```python
from build123d import *

# Parameters (mm, degrees)
ALUMINUM_PLATE_DEPTH            = 3.175
LPATTERN1_COUNT                 = 2
LPATTERN1_PITCH                 = 35
LPATTERN1_COUNT_DIR2            = 2
LPATTERN1_PITCH_DIR2            = 77
CIRPATTERN1_COUNT               = 4
TAP_DRILL_FOR_M5X0_8_TAP1_D     = 4.2
TAP_DRILL_FOR_M5X0_8_TAP1_DEPTH = 25.4
TAP_DRILL_FOR_M5X0_8_TAP1_TIP   = 1.2618073
TAP_DRILL_FOR_8_32_TAP1_D       = 3.4544
TAP_DRILL_FOR_8_32_TAP1_DEPTH   = 12.7
TAP_DRILL_FOR_8_32_TAP1_TIP     = 1.037806461
CUT_EXTRUDE1_DEPTH              = 3.175
CIRPATTERN3_COUNT               = 4
TAP_DRILL_FOR_6_32_TAP1_D       = 2.7051
TAP_DRILL_FOR_6_32_TAP1_DEPTH   = 12.7
TAP_DRILL_FOR_6_32_TAP1_TIP     = 0.81269403


with BuildPart() as part:
    # Sketch2 → Aluminum plate (new body)
    with BuildSketch(Plane(origin=(0, 0, 0), x_dir=(1, 0, 0), z_dir=(0, 1, 0))):
        with BuildLine():
            Line((58.024404898, -30.931736602), (-20.876528813, -30.930973959))
            ThreePointArc((-20.876528813, -30.930973959), (-24.412048563, -29.466473691), (-25.876480484, -25.93092563))
            Line((-25.876480484, -25.93092563), (-25.875595093, 65.669074365))
            ThreePointArc((-25.875595093, 65.669074365), (-24.411094826, 69.204594116), (-20.875546764, 70.669026036))
            Line((-20.875546764, 70.669026036), (58.024501561, 70.668263401))
            ThreePointArc((58.024501561, 70.668263401), (61.560004224, 69.20378022), (63.024453231, 65.668263401))
            Line((63.024453231, 65.668263401), (63.024453227, -25.931736603))
            ThreePointArc((63.024453227, -25.931736603), (61.559970046, -29.467287596), (58.024404898, -30.931736602))
        make_face()
        Polygon((40.164453228, -4.2611466), (-3.015546772, -4.261146598), (-3.01554677, 38.918853402), (40.16445323, 38.9188534), align=None, mode=Mode.SUBTRACT)
    extrude(amount=ALUMINUM_PLATE_DEPTH)

    # Sketch12 → Tap Drill for M3x0.5 Tap1 (revolve, cut)
    with BuildSketch(Plane(origin=(-19.925892409, 3.175, -34.909619628), x_dir=(0, 0, 1), z_dir=(1, 0, 0))):
        Polygon((0, 0), (0, 26.151075774), (1.25, 25.4), (1.25, 0), align=None)
    tap_drill_for_m3x0_5_tap1 = revolve(axis=Axis((-19.925892409, 9.525, -34.909619628), (0, -1, 0)), mode=Mode.SUBTRACT)

    # LPattern1: Tap Drill for M3x0.5 Tap1 2 × 2
    with Locations(*[(j * LPATTERN1_PITCH_DIR2, 0, i * LPATTERN1_PITCH) for i in range(LPATTERN1_COUNT) for j in range(LPATTERN1_COUNT_DIR2) if (i, j) != (0, 0)]):
        add(tap_drill_for_m3x0_5_tap1, mode=Mode.SUBTRACT)

    # Sketch14 → Tap Drill for M3x0.5 Tap2 (revolve, cut)
    with BuildSketch(Plane(origin=(42.384453228, 3.175, -17.329161252), x_dir=(0, 0, 1), z_dir=(1, 0, 0))):
        Polygon((0, 0), (0, 26.151075774), (1.25, 25.4), (1.25, 0), align=None)
    tap_drill_for_m3x0_5_tap2 = revolve(axis=Axis((42.384453228, 9.525, -17.329161252), (0, -1, 0)), mode=Mode.SUBTRACT)

    # CirPattern1: Tap Drill for M3x0.5 Tap2 ×4 about axis
    cirpattern1_axis = Axis((18.574453229, 0, -17.328853401), (0, 1, 0))
    for i in range(1, CIRPATTERN1_COUNT):
        add(tap_drill_for_m3x0_5_tap2.rotate(cirpattern1_axis, i * 360 / CIRPATTERN1_COUNT), mode=Mode.SUBTRACT)

    # Tap Drill for M5x0.8 Tap1
    with Locations(Plane.XZ):
        with Locations((-19.525700823, -54.730512991), (56.674299173, -54.729776455), (56.67357614, 20.073223545), (-19.526423857, 20.072487009)):
            Hole(TAP_DRILL_FOR_M5X0_8_TAP1_D / 2, depth=TAP_DRILL_FOR_M5X0_8_TAP1_DEPTH)
            with Locations((0, 0, -(TAP_DRILL_FOR_M5X0_8_TAP1_DEPTH + TAP_DRILL_FOR_M5X0_8_TAP1_TIP / 2))):  # 118° drill point
                Cone(0, TAP_DRILL_FOR_M5X0_8_TAP1_D / 2, TAP_DRILL_FOR_M5X0_8_TAP1_TIP, mode=Mode.SUBTRACT)

    # Tap Drill for _8-32 Tap1
    with Locations(Plane(origin=(0, 3.175, 0), x_dir=(-1, 0, 0), z_dir=(0, 1, 0))):
        with Locations((-2.699395239, -64.668798164), (-34.449395238, -64.668491274)):
            Hole(TAP_DRILL_FOR_8_32_TAP1_D / 2, depth=TAP_DRILL_FOR_8_32_TAP1_DEPTH)
            with Locations((0, 0, -(TAP_DRILL_FOR_8_32_TAP1_DEPTH + TAP_DRILL_FOR_8_32_TAP1_TIP / 2))):  # 118° drill point
                Cone(0, TAP_DRILL_FOR_8_32_TAP1_D / 2, TAP_DRILL_FOR_8_32_TAP1_TIP, mode=Mode.SUBTRACT)

    # Sketch24 → Cut-Extrude1 (cut)
    with BuildSketch(Plane(origin=(0, 3.175, 0), x_dir=(1, 0, 0), z_dir=(0, 1, 0))):
        with BuildLine():
            Line((21.16445323, 40.9188534), (21.16445323, 44.8563534))
            ThreePointArc((21.16445323, 44.8563534), (21.750239668, 46.270566962), (23.16445323, 46.8563534))
            Line((23.16445323, 46.8563534), (46.101953228, 46.8563534))
            ThreePointArc((46.101953228, 46.8563534), (47.516166791, 46.270566962), (48.101953228, 44.8563534))
            Line((48.101953228, 44.8563534), (48.101953228, 21.9188534))
            ThreePointArc((48.101953228, 21.9188534), (47.516166791, 20.504639837), (46.101953228, 19.9188534))
            Line((46.101953228, 19.9188534), (42.164453228, 19.9188534))
            ThreePointArc((42.164453228, 19.9188534), (40.750239666, 19.333066962), (40.164453228, 17.9188534))
            Line((40.164453228, 17.9188534), (40.164453228, 17.3288534))
            Line((40.164453228, 17.3288534), (18.57445323, 38.9188534))
            Line((18.57445323, 38.9188534), (19.16445323, 38.9188534))
            ThreePointArc((19.16445323, 38.9188534), (20.578666793, 39.504639837), (21.16445323, 40.9188534))
        make_face()
    cut_extrude1 = extrude(amount=-CUT_EXTRUDE1_DEPTH, mode=Mode.SUBTRACT)

    # CirPattern3: Cut-Extrude1 ×4 about axis
    cirpattern3_axis = Axis((18.574453229, 0, -17.328853401), (0, 1, 0))
    for i in range(1, CIRPATTERN3_COUNT):
        add(cut_extrude1.rotate(cirpattern3_axis, i * 360 / CIRPATTERN3_COUNT), mode=Mode.SUBTRACT)

    # Tap Drill for _6-32 Tap1
    with Locations(Plane(origin=(0, 3.175, 0), x_dir=(-1, 0, 0), z_dir=(0, 1, 0))):
        with Locations((-11.032976674, 17.431282391), (-26.114226674, 17.431282391)):
            Hole(TAP_DRILL_FOR_6_32_TAP1_D / 2, depth=TAP_DRILL_FOR_6_32_TAP1_DEPTH)
            with Locations((0, 0, -(TAP_DRILL_FOR_6_32_TAP1_DEPTH + TAP_DRILL_FOR_6_32_TAP1_TIP / 2))):  # 118° drill point
                Cone(0, TAP_DRILL_FOR_6_32_TAP1_D / 2, TAP_DRILL_FOR_6_32_TAP1_TIP, mode=Mode.SUBTRACT)


solid = part.part
```
Work out the finished part from the listing and answer in its coordinate system (mm). Give positions to 0.01 mm unless a question says otherwise; leave off trailing zeros. Loops run counter-clockwise (first coordinate to the right, second up) from the corner with the lowest first, then second, coordinate; pieces in that order, holes last. Notation, with made-up numbers: M -15,48 L 24,48 A29 ccw 24,69 Z; hole C 81.5,53 d6. An arc over 180 degrees is marked long. One line per item, written item: value. Start each with the question number.
1. Determine the mould class of faces 1 (the face through (-24.45, 1.565, -69.166)), 2 (the face through (10.857, 1.565, 18.772)), 3 (the face through (63.024, 2, -21)), 4 (the face through (15.984, 2, -43)) for opening direction Z: released by +Z, released by -Z, zero draft, split by the parting line, or undercut.
2. Find the intervals of material crossed by probe 1 along Z at (x, y) = (-7, 0.65); probe 2 along X at (y, z) = (2.1, -28); probe 3 along Z at (x, y) = (18, 1.55), in increasing order.
3. Each of these flat-tipped pins is pushed along its axis until it touches: P1, Ø2, axis at x = 34.45, z = -64.67, coming from the +Y side; P2, Ø5.5, axis at x = 56.67, z = 20.07, coming from the +Y side (3 decimals). Where does it stop, or does it pass through?
4. Find section C-C (y = 0.7). State how many separate pieces and enclosed holes the cut face has, and give its area (3 significant figures).
5. Find section A-A (z = -30). Give the vertices of the cut face in (x, y) (3 decimals), and give its area (3 significant figures).
Reported:
1. face 1: released by -Z
1. face 2: undercut
1. face 3: zero draft
1. face 4: undercut
2. probe 1: z = -70.67 to -46.86, -19.92 to -14.74, 12.2 to 30.93
2. probe 2: x = -25.88 to -10.95, 48.1 to 63.02
2. probe 3: z = -70.67 to -42.25, -40.03 to -38.92, 4.26 to 5.37, 7.59 to 30.93
3. P1: passes through
3. P2: stops at y = 3.175
4. separate pieces: 1
4. enclosed holes: 17
4. area: 5,570 mm²
5. outline: M -25.876,0 L -10.953,0 L -10.953,3.175 L -25.876,3.175 Z; M 48.102,0 L 63.024,0 L 63.024,3.175 L 48.102,3.175 Z
5. area: 94.8 mm²
